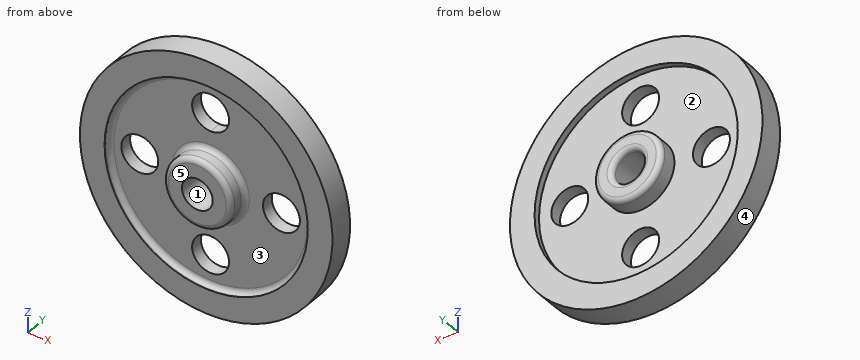
from build123d import *

# Parameters (mm, degrees)
F2_R     = 19.05
F3_DEPTH = 25.4
F4_R     = 5.08
F5_R     = 5.08
F6_R     = 5.08


with BuildPart() as f1:
    # F0 (on Right) → F1 (revolve)
    with BuildSketch(Plane.YZ):
        Polygon((-25.4, 34.902796), (-25.4, 15.852796), (0, 15.852796), (25.4, 15.852796), (25.4, 34.902796), (6.35, 34.902796), (6.35, 104.752796), (12.7, 104.752796), (12.7, 130.152796), (-12.7, 130.152796), (-12.7, 104.752796), (-6.35, 104.752796), (-6.35, 34.902796), align=None)
    revolve(axis=Axis((0, 11.529056, 0), (0, 1, 0)))

    # F2 (on face) → F3 (cut)
    with BuildSketch(Plane(origin=(0, 6.35, 0), x_dir=(-1, 0, 0), z_dir=(0, 1, 0))):
        with BuildLine():
            ThreePointArc((19.05, 73.025), (-13.470384, 86.495384), (0, 53.975))
            ThreePointArc((0, 53.975), (13.470384, 59.554616), (19.05, 73.025))
        make_face()
        with Locations((73.025, 0)):
            Circle(F2_R)
        with Locations((0, -73.025)):
            Circle(F2_R)
        with Locations((-73.025, 0)):
            Circle(F2_R)
    extrude(amount=-F3_DEPTH, mode=Mode.SUBTRACT)

    # F4
    f4_edges = [f1.edges().sort_by_distance(p)[0] for p in [
        (0, -25.4, -34.902796),
        (0, -6.35, -34.902796),
        (0, -15.875, 34.902796),
    ]]
    fillet(f4_edges, radius=F4_R)

    # F5
    f5_edges = [f1.edges().sort_by_distance(p)[0] for p in [
        (0, -6.35, -104.752796),
    ]]
    fillet(f5_edges, radius=F5_R)

    # F6
    f6_edges = [f1.edges().sort_by_distance(p)[0] for p in [
        (0, 25.4, -15.852796),
        (0, 25.4, -34.902796),
    ]]
    fillet(f6_edges, radius=F6_R)


solid = f1.part
The listing builds one solid part. Answer for the finished solid, in the listing's coordinates (mm). Face numbers are marked on the shaded views. A direction names the side the tool comes from. Coordinates: 2 decimals unless noted, no trailing zeros. Write each loop counter-clockwise with the first axis right and the second up, starting at its lowest first coordinate (ties: lowest second). Pieces come first, ordered by that corner, then holes. Notation, with made-up numbers: (44, -2) - (84, -2) arc R35 ccw to (84, 30) - close; hole circle Ø8 at (33, 86.25). An arc over 180 degrees is marked (long way). Put each result on its own line as item: value.
1. A tool of negligible diameter and unlimited length cuts with its end or side. For the marked faces 1 and 2, from which of +Z, -Z, +X, -X, +Y, -Y can it reach the whole face along a straight path? Write none if from no direction.
Answer sheet:
face 1: +Y, -Y
face 2: +Y
2. Determine the mould class of the marked faces 3, 4 and 5 for opening direction Z: pulls with the +Z half, pulls with the -Z half, needs draft (parallel to the pull), parting line crosses it, or undercut.
Answer sheet:
face 3: undercut
face 4: parting line crosses it
face 5: needs draft
3. The part is cut by section C-C on z = 114.5. Give the vertices of the cut face in (x, y).
Answer sheet:
outline: (-61.88, -12.7) - (61.88, -12.7) - (61.88, 12.7) - (-61.88, 12.7) - close
4. The part is cut by section A-A on y = 9.5. Give the vertices of the cut face in (x, z), plus the area to 3 significant figures.
Answer sheet:
outline: circle Ø260.31 at (0, 0); circle Ø69.81 at (0, 0); hole circle Ø209.51 at (0, 0); hole circle Ø31.71 at (0, 0)
area: 21,800 mm^2
5. Flat-ended cylindrical pins translate along their axes: pin 1 Ø1 at (x, y) = (102, 11) entering from +Z; pin 2 Ø3 at (x, y) = (48.5, -11) entering from +Z; pin 3 Ø12 at (x, y) = (17.5, 15) entering from +Z. Find the tip coordinate at first contact, or state that the pin passes through.
Answer sheet:
pin 1: stops at z = 81.47
pin 2: stops at z = 121.37
pin 3: stops at z = 129.6
6. Find the intervals of material crossed by line 1 along X through (y, z) = (-12, 0); line 2 along X through (y, z) = (8, 18); line 3 along X through (y, z) = (-13, 0), in increasing order. Write a range as from..to.
Answer sheet:
line 1: x = -130.15..-104.75, -34.9..-15.85, 15.85..34.9, 104.75..130.15
line 2: x = -128.9..-103.19, -29.9..29.9, 103.19..128.9
line 3: x = -34.9..-15.85, 15.85..34.9
7. The part is cut by section B-B on z = 0. State how many separate pieces and enclosed holes the cut face has, plus the area to 3 significant figures.
Answer sheet:
separate pieces: 4
enclosed holes: 0
area: 4,020 mm^2
